Here's the drawing with two shaded views (mm, measured from the low corner). I have some questions. A direction names the side the tool comes from. Give positions to 0.01 mm unless a question says otherwise; leave off trailing zeros. Loops run counter-clockwise (first coordinate to the right, second up) from the corner with the lowest first, then second, coordinate; pieces in that order, holes last. Notation, with made-up numbers: M 39,30.5 L 57,30.5 A18 ccw 57,45.5 Z; hole C -20.5,-12 d7. An arc over 180 degrees is marked long. Use a Markdown table: item, result. Add a question column.
1) Suppose I cut it at C-C on y = 170. List the corners of the cut face in (x, z) for me, and give its area (3 significant figures).
2) If I drill on line 1 along X through (y, z) = (50, 27.5); line 2 along X through (y, z) = (185, 81); line 3 along Z through (x, y) = (194.5, 160.5), over which ranges is the centre line in solid material (lowest first)? Write a range as [from, to].
3) We'd pull the mould along X, two halves only. Please class the marked faces 1, 2, 3 and 4: +X half, -X half, draft (parallel to the pull), parting line (faces both ways), or undercut.
4) Suppose I cut it at D-D on x = 140. List the corners of the cut face in (y, z) for me, and give its area (3 significant figures).
5) Suppose I cut it at A-A on y = 61.5. List the corners of the cut face in (x, z) for me.
6) Which directions (+Z, -Z, +X, -X, +Y, -Y) give clear straight access to the entire face, cutting with the end or side of a thin tool? Please do the marked faces 5, 6 and 7.
7) Will these pins go through, and if not, where does the flat tip stop? pin 1 Ø20 at (x, y) = (108.5, 177.5) entering from -Z; pin 2 Ø3 at (x, y) = (1.5, 63.5) entering from +Z; pin 3 Ø16 at (y, z) = (81, 22.5) entering from -X; pin 4 Ø4.5 at (y, z) = (170.5, 94) entering from +X.
8) Suppose I cut it at B-B on z = 85.5. List the corners of the cut face in (x, y) for me, and give its area (3 significant figures).
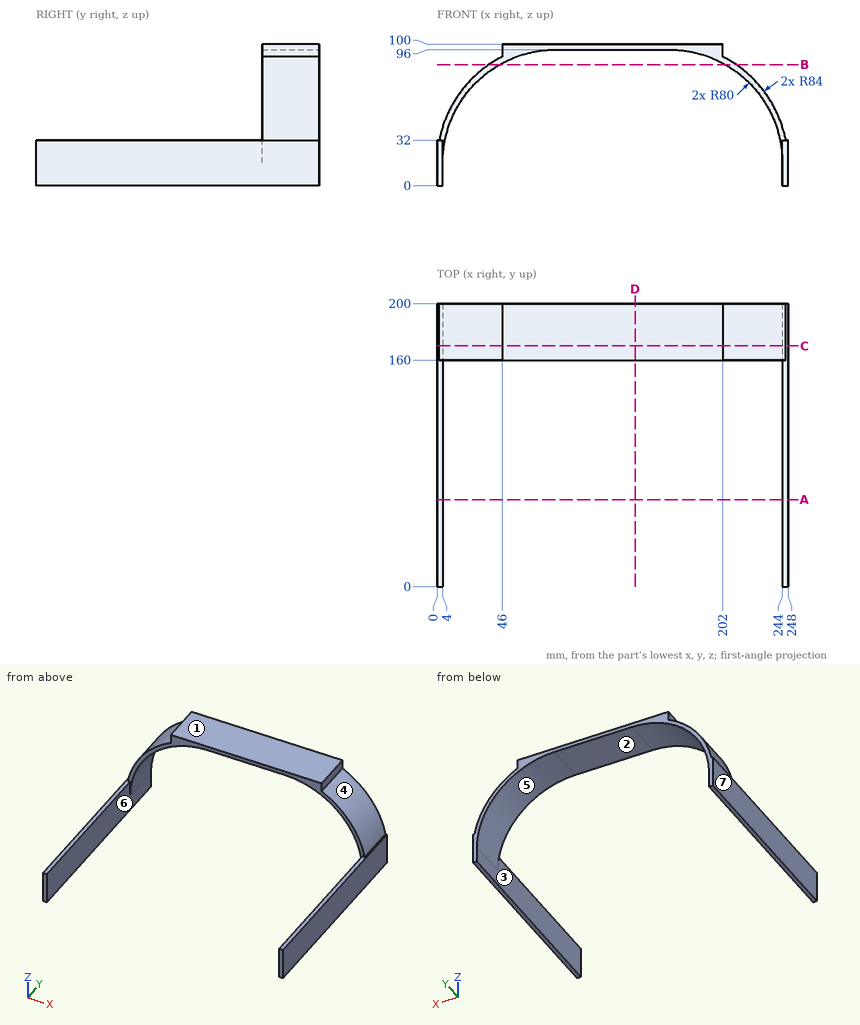
Answer block:
| question | item | result |
|---|---|---|
| 1 | outline | M 0,0 L 4,0 L 4,16 A80 cw 84,96 L 164,96 A80 cw 244,16 L 244,0 L 248,0 L 248,32 L 246.46,32 A84 ccw 202,90.91 L 202,100 L 46,100 L 46,90.91 A84 ccw 1.54,32 L 0,32 Z |
| 1 | area | 1,720 mm^2 |
| 2 | line 1 | x = [0, 4], [244, 248] |
| 2 | line 2 | x = [30.79, 37.36], [210.64, 217.21] |
| 2 | line 3 | z = [89.96, 100] |
| 3 | face 1 | draft |
| 3 | face 2 | undercut |
| 3 | face 3 | undercut |
| 3 | face 4 | +X half |
| 4 | outline | M 160,96 L 200,96 L 200,100 L 160,100 Z |
| 4 | area | 160 mm^2 |
| 5 | outline | M 0,0 L 4,0 L 4,32 L 0,32 Z; M 244,0 L 248,0 L 248,32 L 244,32 Z |
| 6 | face 5 | -Z, +Y, -Y |
| 6 | face 6 | -Z, -Y |
| 6 | face 7 | +Z, -Z, -X, +Y, -Y |
| 7 | pin 1 | stops at z = 96 |
| 7 | pin 2 | stops at z = 32 |
| 7 | pin 3 | stops at x = 0 |
| 7 | pin 4 | stops at x = 202 |
| 8 | outline | M 36.82,160 L 44.38,160 L 44.38,200 L 36.82,200 Z; M 203.62,160 L 211.18,160 L 211.18,200 L 203.62,200 Z |
| 8 | area | 605 mm^2 |
